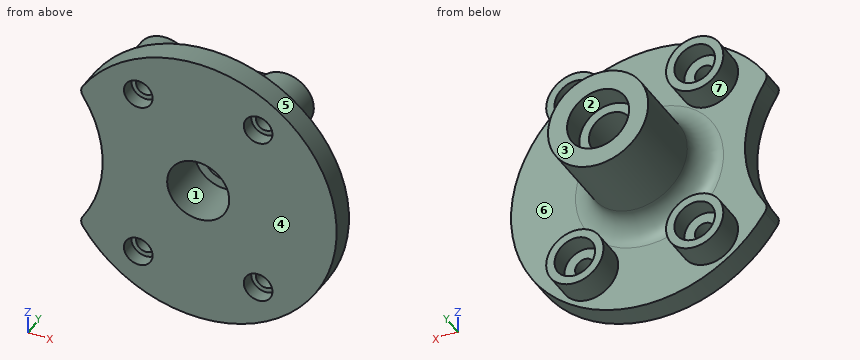
from build123d import *

# Parameters (mm, degrees)
ESQUISSE3_R             = 6.5
BOSS_EXTRU_1_DEPTH      = 5
CONG_1_R                = 5
ESQUISSE5_R             = 6
ESQUISSE5_R_2           = 4.25
BOSS_EXTRU_3_DEPTH      = 6
ESQUISSE8_R             = 4.25
BOSS_EXTRU_4_DEPTH      = 2
ESQUISSE6_R             = 2
ENL_V_MAT_EXTRU_1_DEPTH = 47.030533345
ESQUISSE7_R             = 3
ENL_V_MAT_EXTRU_2_DEPTH = 3
CONG_2_R                = 2


with BuildPart() as part:
    # Esquisse2 → Révolution1 (revolve)
    with BuildSketch(Plane(origin=(0, 0, 0), x_dir=(0, 0, -1), z_dir=(1, 0, 0))):
        Polygon((6.5, 5), (6.5, 10), (10.5, 10), (10.5, -10.9), (6.5, -10.9), (6.5, -5), (4.5, -5), (4.5, 0), (4.5, 5), align=None)
    revolve(axis=Axis((0, 0, 0), (0, 1, 0)))

    # Esquisse3 → Boss.-Extru.1 (add)
    with BuildSketch(Plane(origin=(0, -10.9, 0), x_dir=(1, 0, 0), z_dir=(0, 1, 0))):
        with BuildLine():
            ThreePointArc((-24.9, 14.865732407), (-20, 0), (-24.9, -14.865732407))
            ThreePointArc((-24.9, -14.865732407), (29, 0), (-24.9, 14.865732407))
        make_face()
        with Locations(Location((0, 0, 0), (0, 0, 90))):
            Circle(ESQUISSE3_R, mode=Mode.SUBTRACT)
    extrude(amount=-BOSS_EXTRU_1_DEPTH)

    # Congé1
    cong_1_edges = [part.edges().sort_by_distance(p)[0] for p in [
        (0, -10.9, 10.5),
    ]]
    fillet(cong_1_edges, radius=CONG_1_R)

    # Esquisse5 → Boss.-Extru.3 (add)
    # profile 1 of 2: a face of its own
    with BuildSketch(Plane(origin=(0, -10.9, 0), x_dir=(1, 0, 0), z_dir=(0, 1, 0))):
        with Locations(Location((-12.550755593, 17.998053071, 0), (0, 0, 90))):
            Circle(ESQUISSE5_R)
        with Locations(Location((-12.550755593, 17.998053071, 0), (0, 0, 270))):
            Circle(ESQUISSE5_R_2, mode=Mode.SUBTRACT)
    # profile 2 of 2: a face of its own
    with BuildSketch(Plane(origin=(0, -10.9, 0), x_dir=(1, 0, 0), z_dir=(0, 1, 0))):
        with Locations(Location((-12.550755593, -17.998053071, 0), (0, 0, 90))):
            Circle(ESQUISSE5_R)
        with Locations(Location((-12.550755593, -17.998053071, 0), (0, 0, 90))):
            Circle(ESQUISSE5_R_2, mode=Mode.SUBTRACT)
    boss_extru_3 = extrude(amount=BOSS_EXTRU_3_DEPTH)

    # Esquisse8 → Boss.-Extru.4 (add)
    with BuildSketch(Plane(origin=(0, -10.9, 0), x_dir=(1, 0, 0), z_dir=(0, 1, 0))):
        with Locations(Location((-12.550755593, -17.998053071, 0), (0, 0, 90))):
            Circle(ESQUISSE8_R)
        with Locations(Location((-12.550755593, 17.998053071, 0), (0, 0, 270))):
            Circle(ESQUISSE8_R)
    boss_extru_4 = extrude(amount=BOSS_EXTRU_4_DEPTH)

    # Esquisse6 → Enlèv. mat.-Extru.1 (cut, symmetric)
    with BuildSketch(Plane(origin=(0, -10.9, 0), x_dir=(1, 0, 0), z_dir=(0, 1, 0))):
        with Locations(Location((-12.550755593, -17.998053071, 0), (0, 0, 270))):
            Circle(ESQUISSE6_R)
        with Locations(Location((-12.550755593, 17.998053071, 0), (0, 0, 270))):
            Circle(ESQUISSE6_R)
    enl_v_mat_extru_1 = extrude(amount=ENL_V_MAT_EXTRU_1_DEPTH, both=True, mode=Mode.SUBTRACT)

    # Esquisse7 → Enlèv. mat.-Extru.2 (cut)
    with BuildSketch(Plane.XZ.offset(15.9)):
        with Locations(Location((-12.550755593, 17.998053071, 0), (0, 0, 270))):
            Circle(ESQUISSE7_R)
        with Locations(Location((-12.550755593, -17.998053071, 0), (0, 0, 270))):
            Circle(ESQUISSE7_R)
    enl_v_mat_extru_2 = extrude(amount=-ENL_V_MAT_EXTRU_2_DEPTH, mode=Mode.SUBTRACT)

    # Congé2
    cong_2_edges = [part.edges().sort_by_distance(p)[0] for p in [
        (-24.9, -13.4, -14.865732407),
        (-24.9, -13.4, 14.865732407),
    ]]
    fillet(cong_2_edges, radius=CONG_2_R)

    # Symétrie1: Boss.-Extru.3, Boss.-Extru.4, Enlèv. mat.-Extru.1, Enlèv. mat.-Extru.2 across plane
    add(boss_extru_3.mirror(Plane(origin=(0, 0, 0), x_dir=(0, 0, 1), z_dir=(1, 0, 0))))
    add(boss_extru_4.mirror(Plane(origin=(0, 0, 0), x_dir=(0, 0, 1), z_dir=(1, 0, 0))))
    add(enl_v_mat_extru_1.mirror(Plane(origin=(0, 0, 0), x_dir=(0, 0, 1), z_dir=(1, 0, 0))), mode=Mode.SUBTRACT)
    add(enl_v_mat_extru_2.mirror(Plane(origin=(0, 0, 0), x_dir=(0, 0, 1), z_dir=(1, 0, 0))), mode=Mode.SUBTRACT)


solid = part.part
CAD build for the part. Positions are in the model's coordinates, mm. Face numbers are marked on the shaded views. A direction names the side the tool comes from. Round coordinates to 2 decimals unless told otherwise and drop trailing zeros. Loops run counter-clockwise (first coordinate to the right, second up) from the corner with the lowest first, then second, coordinate; pieces in that order, holes last.
(1) Cut at B-B (z = 0). Give the cut face in (x, y), plus the area to 3 significant figures.
(2) Drop flat-ended pins along their axis: pin 1 (5.5 mm diameter, centred on x = 12.55, z = -18, fed in from +Y); pin 2 (3 mm diameter, centred on x = -12.55, z = -18, fed in from -Y); pin 3 (6 mm diameter, centred on x = -15, z = 19.5, fed in from +Y); pin 4 (1 mm diameter, centred on x = 5, y = -8.5, fed in from -Z). Give the stop position or say it passes through.
(3) Two-plate mould, pull along Z, no slides. Class the marked faces 4, 5, 6 and 7: +Z half, -Z half, draft (parallel to the pull), parting line (faces both ways), or undercut.
(4) Cut at D-D (x = -21). Give the cut face in (y, z).
(5) Cut at A-A (x = 0). Give the cut face in (y, z).
(6) Wall check: line 1 along X through (y, z) = (7.8, 0); line 2 along Y through (x, z) = (-4, 3); line 3 along Y through (x, z) = (-17.5, 15). Give the ranges that are in metal, low to high.
(7) Cut at C-C (y = 7.5). Give the cut face in (x, z), plus the area to 3 significant figures.
(8) Which spindle directions (+Z, -Z, +X, -X, +Y, -Y) get a long thin tool onto all of the face, cutting with end or side? Do the marked faces 1, 2 and 3. Say none if no direction does.
Findings below:
1. outline: (-20, -15.9) - (-6.5, -15.9) - (-6.5, -5) - (-4.5, -5) - (-4.5, 5) - (-6.5, 5) - (-6.5, 10) - (-10.5, 10) - (-10.5, -5.9) arc R5 cw to (-15.5, -10.9) - (-20, -10.9) - close; (4.5, -5) - (6.5, -5) - (6.5, -15.9) - (29, -15.9) - (29, -10.9) - (15.5, -10.9) arc R5 cw to (10.5, -5.9) - (10.5, 10) - (6.5, 10) - (6.5, 5) - (4.5, 5) - close
1. area: 398 mm2
2. pin 1: stops at y = -8.9
2. pin 2: passes through
2. pin 3: stops at y = -4.9
2. pin 4: stops at z = -10.5
3. face 4: draft
3. face 5: parting line
3. face 6: undercut
3. face 7: undercut
4. outline: (-15.9, -20) - (-10.9, -20) - (-10.9, -7) - (-15.9, -7) - close; (-15.9, 7) - (-10.9, 7) - (-10.9, 20) - (-15.9, 20) - close
5. outline: (-15.9, -29) - (-10.9, -29) - (-10.9, -15.5) arc R5 cw to (-5.9, -10.5) - (10, -10.5) - (10, -6.5) - (5, -6.5) - (5, -4.5) - (-5, -4.5) - (-5, -6.5) - (-15.9, -6.5) - close; (-15.9, 6.5) - (-5, 6.5) - (-5, 4.5) - (5, 4.5) - (5, 6.5) - (10, 6.5) - (10, 10.5) - (-5.9, 10.5) arc R5 cw to (-10.9, 15.5) - (-10.9, 29) - (-15.9, 29) - close
6. line 1: x = -10.5 to -6.5, 6.5 to 10.5
6. line 2: y = -5 to 5
6. line 3: y = -15.9 to -4.9
7. outline: circle Ø21 at (0, 0); hole circle Ø13 at (0, 0)
7. area: 214 mm2
8. face 1: -Y
8. face 2: +Y
8. face 3: +Z, -Z, +X, -X, +Y
